from build123d import *

# Parameters (mm, degrees)
F0_W     = 80
F0_H     = 12.7
F1_DEPTH = 12.7
F3_D     = 10
F5_D     = 4.4
F7_D     = 5.5


with BuildPart() as f1:
    # F0 (on Front) → F1 (new body)
    with BuildSketch(Plane.XZ):
        Rectangle(F0_W, F0_H)
    extrude(amount=F1_DEPTH)

    # F3 (through all)
    with Locations(Plane.XZ.offset(12.7)):
        with Locations((-4, 0), (4, 0)):
            Hole(F3_D / 2)

    # F5 (through all)
    with Locations(Plane.XY.offset(6.35)):
        with Locations((20, -6.0262801126), (35, -6.0262801126)):
            Hole(F5_D / 2)

    # F7 (through all)
    with Locations(Plane.XY.offset(6.35)):
        with Locations((-35, -6.3651315868), (-20, -6.3651315868)):
            Hole(F7_D / 2)


solid = f1.part
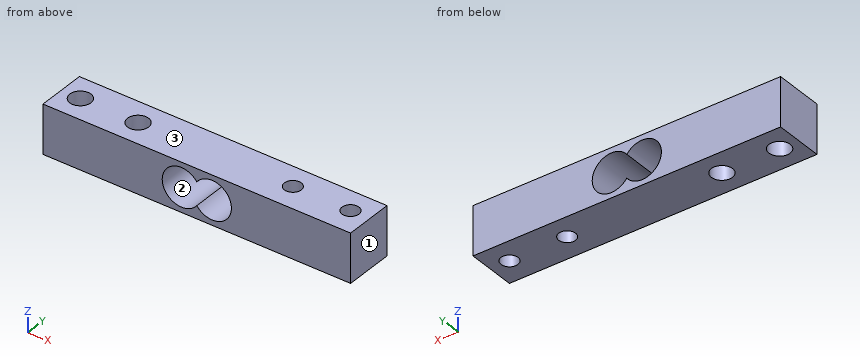
Work out the finished part from the listing and answer in its coordinate system (mm). Face numbers are marked on the shaded views. Round coordinates to 2 decimals unless told otherwise and drop trailing zeros. Write each loop counter-clockwise with the first axis right and the second up, starting at its lowest first coordinate (ties: lowest second). Pieces come first, ordered by that corner, then holes. Notation, with made-up numbers: (-34.5, 11.25) -> (9.5, 11.25) arc R37 cw to (9.5, 47.25) -> close; hole circle Ø9 at (-38, 76). An arc over 180 degrees is marked (long way). Answer as CSV lines item,"result". Start each with the question number.
(1) The part is cut by section D-D, the plane z = -4. Give the vertices of the cut face in (x, y).
(2) Find the intervals of material crossed by probe 1 along X at (y, z) = (-6.5, -1.5); probe 2 along X at (y, z) = (-8.5, 2); probe 3 along Z at (x, y) = (-4, -3.25), in increasing order.
(3) The part is cut by section B-B, the plane z = 0.5. Give the vertices of the cut face in (x, y), then the cut area to 3 significant figures.
(4) The part is cut by section C-C, the plane y = -0.75. Give the vertices of the cut face in (x, z).
(5) Each of these flat-tipped pins is pushed along its axis until it touches: pin 1 (4 mm diameter, centred on x = -24, z = 4, fed in from +Y); pin 2 (4.5 mm diameter, centred on x = -20, y = -6.37, fed in from -Z). Where does it stop, or does it pass through?
(6) The mould has two halves that part along Z. Classify the marked faces 1, 2 and 3: +Z half, -Z half, draft (parallel to the pull), parting line (faces both ways), or undercut.
(7) The part is cut by section A-A, the plane x = 35. Give the vertices of the cut face in (y, z), then the cut area to 3 significant figures.
Output values:
1,outline,"(-40, -12.7) -> (-7, -12.7) -> (-7, 0) -> (-40, 0) -> close; (-1, -12.7) -> (1, -12.7) -> (1, 0) -> (-1, 0) -> close; (7, -12.7) -> (40, -12.7) -> (40, 0) -> (7, 0) -> close; hole circle Ø5.5 at (-35, -6.37); hole circle Ø5.5 at (-20, -6.37); hole circle Ø4.4 at (20, -6.03); hole circle Ø4.4 at (35, -6.03)"
2,probe 1,"x = -40 to -37.75, -32.25 to -22.75, -17.25 to -8.77, 8.77 to 17.85, 22.15 to 32.85, 37.15 to 40"
2,probe 2,"x = -40 to -36.73, -33.27 to -21.73, -18.27 to -8.58, 8.58 to 40"
2,probe 3,"z = -6.35 to -5, 5 to 6.35"
3,outline,"(-40, -12.7) -> (-8.97, -12.7) -> (-8.97, 0) -> (-40, 0) -> close; (8.97, -12.7) -> (40, -12.7) -> (40, 0) -> (8.97, 0) -> close; hole circle Ø5.5 at (-35, -6.37); hole circle Ø5.5 at (-20, -6.37); hole circle Ø4.4 at (20, -6.03); hole circle Ø4.4 at (35, -6.03)"
3,area,"710 mm²"
4,outline,"(-40, -6.35) -> (40, -6.35) -> (40, 6.35) -> (-40, 6.35) -> close; hole (0, -3) arc R5 ccw (long way) to (0, 3) arc R5 ccw (long way) to start"
5,pin 1,"stops at y = 0"
5,pin 2,"passes through"
6,face 1,"draft"
6,face 2,"undercut"
6,face 3,"+Z half"
7,outline,"(-12.7, -6.35) -> (-8.23, -6.35) -> (-8.23, 6.35) -> (-12.7, 6.35) -> close; (-3.83, -6.35) -> (0, -6.35) -> (0, 6.35) -> (-3.83, 6.35) -> close"
7,area,"105 mm²"
